from build123d import *

# Parameters (mm, degrees)
SALIENTE_EXTRUIR1_DEPTH = 20
SALIENTE_EXTRUIR2_DEPTH = 5
SKETCH1_R               = 12
BOSS_EXTRUDE1_DEPTH     = 11
SKETCH2_R               = 12.5
BOSS_EXTRUDE2_DEPTH     = 3
FILLET1_R               = 2
CUT_EXTRUDE2_DEPTH      = 15
SKETCH7_R               = 15
CUT_EXTRUDE3_DEPTH      = 28


with BuildPart() as part:
    # Croquis1 → Saliente-Extruir1 (new body)
    with BuildSketch(Plane(origin=(0, 0, 0), x_dir=(1, 0, 0), z_dir=(0, 1, 0))):
        with BuildLine():
            Line((-57.44056846, 112.613636364), (-62.4354005, 2.840909091))
            ThreePointArc((-62.4354005, 2.840909091), (0, -62.5), (62.4354005, 2.840909091))
            Line((62.4354005, 2.840909091), (57.44056846, 112.613636364))
            ThreePointArc((57.44056846, 112.613636364), (47.362244362, 142.604720655), (22.943989921, 162.724029877))
            ThreePointArc((22.943989921, 162.724029877), (20.757274923, 164.567893199), (19.93911948, 167.308728127))
            Line((19.93911948, 167.308728127), (19.93911948, 203.118676651))
            ThreePointArc((19.93911948, 203.118676651), (18.474653385, 206.654210557), (14.93911948, 208.118676651))
            Line((14.93911948, 208.118676651), (-15.06088052, 208.118676651))
            ThreePointArc((-15.06088052, 208.118676651), (-18.596414426, 206.654210557), (-20.06088052, 203.118676651))
            Line((-20.06088052, 203.118676651), (-20.06088052, 167.255587217))
            ThreePointArc((-20.06088052, 167.255587217), (-20.876125318, 164.519198375), (-23.056010079, 162.675140239))
            ThreePointArc((-23.056010079, 162.675140239), (-47.396870484, 142.554364812), (-57.44056846, 112.613636364))
        make_face()
        with BuildLine():
            Line((-52.44573642, 112.386363636), (-57.44056846, 2.613636364))
            ThreePointArc((-57.44056846, 2.613636364), (0, -57.5), (57.44056846, 2.613636364))
            Line((57.44056846, 2.613636364), (52.44573642, 112.386363636))
            ThreePointArc((52.44573642, 112.386363636), (0, 162.5), (-52.44573642, 112.386363636))
        make_face(mode=Mode.SUBTRACT)
    extrude(amount=SALIENTE_EXTRUIR1_DEPTH)



with BuildPart() as body_2:
    # Croquis2 → Saliente-Extruir2 (new body)
    with BuildSketch(Plane(origin=(0, 0, 0), x_dir=(-1, 0, 0), z_dir=(0, -1, 0))):
        with BuildLine():
            Line((5, 83.229490169), (5, 16.770509831))
            ThreePointArc((5, 16.770509831), (15.80191276, 7.519943692), (16.167891819, -6.696960066))
            Line((16.167891819, -6.696960066), (53.123073119, -22.004297361))
            ThreePointArc((53.123073119, -22.004297361), (50.429243253, -27.625014479), (47.142858448, -32.921131471))
            Line((47.142858448, -32.921131471), (6.696960066, -16.167891819))
            ThreePointArc((6.696960066, -16.167891819), (0, -17.5), (-6.696960066, -16.167891819))
            Line((-6.696960066, -16.167891819), (-47.142858448, -32.921131471))
            ThreePointArc((-47.142858448, -32.921131471), (-50.429243253, -27.625014479), (-53.123073119, -22.004297361))
            Line((-53.123073119, -22.004297361), (-16.167891819, -6.696960066))
            ThreePointArc((-16.167891819, -6.696960066), (-15.80191276, 7.519943692), (-5, 16.770509831))
            Line((-5, 16.770509831), (-5, 83.229490169))
            ThreePointArc((-5, 83.229490169), (-15.80191276, 92.480056308), (-16.167891819, 106.696960066))
            Line((-16.167891819, 106.696960066), (-51.282274043, 121.241813418))
            ThreePointArc((-51.282274043, 121.241813418), (-49.596532898, 127.217256589), (-47.217157465, 132.951907131))
            Line((-47.217157465, 132.951907131), (-6.696960066, 116.167891819))
            ThreePointArc((-6.696960066, 116.167891819), (0, 117.5), (6.696960066, 116.167891819))
            Line((6.696960066, 116.167891819), (47.217157465, 132.951907131))
            ThreePointArc((47.217157465, 132.951907131), (49.596532898, 127.217256589), (51.282274043, 121.241813418))
            Line((51.282274043, 121.241813418), (16.167891819, 106.696960066))
            ThreePointArc((16.167891819, 106.696960066), (15.80191276, 92.480056308), (5, 83.229490169))
        make_face()
    extrude(amount=-SALIENTE_EXTRUIR2_DEPTH)


with BuildPart() as part_1:
    add(part.part)

    add(body_2.part)  # Boss-Extrude1 merges body 2
    # Sketch1 → Boss-Extrude1 (add)
    with BuildSketch(Plane(origin=(0, 5, 0), x_dir=(1, 0, 0), z_dir=(0, 1, 0))):
        with Locations(Location((0, 100, 0), (0, 0, 90))):
            Circle(SKETCH1_R)
        with Locations(Location((0, 0, 0), (0, 0, 90))):
            Circle(SKETCH1_R)
    extrude(amount=BOSS_EXTRUDE1_DEPTH)

    # Sketch2 → Boss-Extrude2 (add)
    with BuildSketch(Plane(origin=(0, 16, 0), x_dir=(1, 0, 0), z_dir=(0, 1, 0))):
        with Locations(Location((0, 100, 0), (0, 0, 270))):
            Circle(SKETCH2_R)
        with Locations(Location((0, 0, 0), (0, 0, 270))):
            Circle(SKETCH2_R)
    extrude(amount=BOSS_EXTRUDE2_DEPTH)

    # Fillet1
    fillet1_edges = [part_1.edges().sort_by_distance(p)[0] for p in [
        (0, 19, -112.5),
        (0, 19, -12.5),
    ]]
    fillet(fillet1_edges, radius=FILLET1_R)

    # Sketch6 → Cut-Extrude2 (cut)
    with BuildSketch(Plane(origin=(0, 19, 0), x_dir=(1, 0, 0), z_dir=(0, 1, 0))):
        Polygon((-10.514481664, 108.393161321), (-2.121320344, 100), (-2.121320344, 87.230677616), (2.121320344, 87.230677616), (2.121320344, 100), (10.425393612, 108.304073268), (8.270497601, 110.391817945), (0, 102.121320344), (-8.354488758, 110.475809101), align=None)
        Polygon((-2.121320344, 12.769322384), (2.121320344, 12.769322384), (2.121320344, 0), (10.425393612, -8.304073268), (8.270497601, -10.391817945), (0, -2.121320344), (-8.354488758, -10.475809101), (-10.514481664, -8.393161321), (-2.121320344, 0), align=None)
    extrude(amount=-CUT_EXTRUDE2_DEPTH, mode=Mode.SUBTRACT)

    # Sketch7 → Cut-Extrude3 (cut)
    with BuildSketch(Plane(origin=(0, 20, 0), x_dir=(1, 0, 0), z_dir=(0, 1, 0))):
        with Locations(Location((-0.03044026, 185.309338326, 0), (0, 0, 270))):
            Circle(SKETCH7_R)
    extrude(amount=-CUT_EXTRUDE3_DEPTH, mode=Mode.SUBTRACT)


solid = part_1.part
CAD build for the part. Positions are in the model's coordinates, mm. A direction names the side the tool comes from. Give positions to 0.01 mm unless a question says otherwise; leave off trailing zeros. Loops run counter-clockwise (first coordinate to the right, second up) from the corner with the lowest first, then second, coordinate; pieces in that order, holes last. Notation, with made-up numbers: M 25.25,35 L 79.25,35 A32 cw 79.25,74 Z; hole C -28.5,-31 d6. An arc over 180 degrees is marked long. Write each question's results on one line, items separated by ' | '.
Q1. Band-saw the part on B-B on y = 9.25. Give the number of separate pieces and of enclosed holes in the cut face, and give its area (3 significant figures).
Geometry check:
separate pieces: 7 | enclosed holes: 2 | area: 4,530 mm²
Q2. Which spindle directions (+Z, -Z, +X, -X, +Y, -Y) get a long thin tool onto all of the face, cutting with end or side? Do faces 1 (the face through (-15.713, 2.465, -7.705)), 2 (the face through (2.121, 12, -6)), 3 (the face through (11.6, 16, -3.8)). Say none if no direction does.
Geometry check:
face 1: +Y, -Y | face 2: +Y | face 3: none
Q3. Mould opens along X. For faces 4 (the face through (19.939, 10, -185)), 5 (the face through (6, 19, -2)), 6 (the face through (11.6, 16.49, -95.34)), 7 (the face through (-20.854, 9.86, -164.553)) say: pulls with the +X half, pulls with the -X half, needs draft (parallel to the pull), parting line crosses it, or undercut.
Geometry check:
face 4: pulls with the +X half | face 5: undercut | face 6: undercut | face 7: pulls with the -X half
Q4. Flat gauge pins, fed straight in: P1, Ø4, axis at y = 11.5, z = -93, coming from the -X side; P2, Ø6.5, axis at x = -1, z = -3, coming from the +Y side; P3, Ø10, axis at y = 9, z = -191, coming from the +X side; P4, Ø8.5, axis at x = 8, z = -100.5, coming from the -Y side. Where does each tip first touch, or does it go through?
Geometry check:
P1: stops at x = -58.42 | P2: stops at y = 19 | P3: stops at x = 19.94 | P4: stops at y = 0
Q5. Band-saw the part on C-C on x = 30.5. Write the cut outline in (y, z).
Geometry check:
outline: M 0,-158.74 L 20,-158.74 L 20,-152.73 L 0,-152.73 Z; M 0,-126.03 L 5,-126.03 L 5,-112.63 L 0,-112.63 Z; M 0,12.63 L 5,12.63 L 5,26.03 L 0,26.03 Z; M 0,48.74 L 20,48.74 L 20,54.55 L 0,54.55 Z
Q6. Probe probe 1 along Z at (x, y) = (1, 10.5); probe 2 along Z at (x, y) = (-11, 17.5); probe 3 along X at (y, z) = (1, 14.5). List the from-to ranges inside material, lowest first.
Geometry check:
probe 1: z = -208.12 to -200.27, -170.34 to -162.49, -111.96 to -103.12, 3.12 to 11.96, 57.49 to 62.49 | probe 2: z = -208.12 to -195.54, -175.08 to -161.33, -105.8 to -94.2, -5.8 to 5.8, 56.44 to 61.52 | probe 3: x = -60.79 to -55.64, -35.01 to 35.01, 55.64 to 60.79
Q7. Band-saw the part on A-A on x = -37.5. Write the cut outline in (y, z), and give its area (3 significant figures).
Geometry check:
outline: M 0,-153.59 L 20,-153.59 L 20,-146.74 L 0,-146.74 Z; M 0,-128.93 L 5,-128.93 L 5,-115.53 L 0,-115.53 Z; M 0,15.53 L 5,15.53 L 5,28.93 L 0,28.93 Z; M 0,43.59 L 20,43.59 L 20,50 L 0,50 Z | area: 399 mm²
